Autodesk Inventor part; units mm, degrees
ref_plane "Work Plane1" through (-7.9612, 0, 0) normal (0, -0.866, -0.5) x (1, 0, 0)
ref_plane "YZ Plane" through (0, 0, 0) normal (1, 0, 0) x (0, 1, 0)
ref_plane "XZ Plane" through (0, 0, 0) normal (0, 1, 0) x (-1, 0, 0)
sketch "Sketch1" plane through (0, 0, 0) normal (1, 0, 0) x (0, 1, 0)
  line L0 (-4.0415, 0) -> (-2.0207, 3.5)
  line L1 (-2.0207, 3.5) -> (2.0207, 3.5)
  line L2 (2.0207, 3.5) -> (4.0415, 0)
  line L3 (4.0415, 0) -> (2.0207, -3.5)
  line L4 (2.0207, -3.5) -> (-2.0207, -3.5)
  line L5 (-2.0207, -3.5) -> (-4.0415, 0)
  point P0 (0, 0)
  point P1 (0, 0)
  dimension "d0" = 8.0829
extrude "Body" add sketch "Sketch1" along normal blind 3.2
sketch "Sketch2" plane through (0, 0, 0) normal (0, 0, 1) x (1, 0, 0)
  line L0 (0, 2.0207) -> (0, 4.0415)
  line L1 (0, 4.0415) -> (3.2, 4.0415)
  line L2 (3.2, 2.0207) -> (3.2, 4.0415)
  line L3 (-0.64, 0) -> (3.84, 0)
  line L4 (0.2525, 4.0415) -> (0, 3.5)
  line L5 (2.9475, 4.0415) -> (3.2, 3.5)
  dimension "d3" = 25
  dimension "d4" = 25
  dimension "d5" = 7
  dimension "d6" = 7
revolve "Chamfer1" cut sketch "Sketch2" angle 360 about axis through (-10, 0, 0) along (1, 0, 0)
sketch "Sketch3" plane through (3.2, 0, 0) normal (1, 0, 0) x (0, 0, -1)
  arc A0 (-1.75, -3.0311) -> (1.75, -3.0311) centre (0, 0) ccw
hole "Thread" at (3.2, 0, 0) direction (-1, 0, 0) diameter 3.242 end through all
chamfer "Chamfer2" distance 0.3789 angle 30 1 edges at (3.2, 0, 1.621) measured on face at (3.2, 2.8569, -0.0651)
chamfer "Chamfer3" distance 0.3789 angle 30 1 edges at (0, 0, 1.621) measured on face at (0, 2.8569, -0.0651)
ref_plane "Work Plane1" through (-7.9612, 0, 0) normal (0, -0.866, -0.5) x (1, 0, 0)
equation "\"d0\" = 1.1547 * SW"
equation "\"d1\" = KOH"
equation "\"d8\" = -0.5 * GD1 + 0.5 * NND"
equation "\"d40\" = -0.5 * GD1 + 0.5 * NND"
equation "\"d10\" = -0.5 * GD1 + 0.5 * NND"
equation "\"d41\" = -0.5 * GD1 + 0.5 * NND"
equation "\"d3\" = ANG1"
equation "\"d4\" = ANG2"
equation "\"d5\" = SW0"
equation "\"d6\" = SW01"
equation "\"ANG1\" = 25deg"
equation "\"ANG2\" = 25deg"
equation "\"NND\" = 4"
equation "\"KOH\" = 3.2"
equation "\"SW\" = 7"
equation "\"SW0\" = SW"
equation "\"SW01\" = SW"
equation "\"GUL\" = 0.541266 * PTC"
equation "\"THREADDIA\" = 4"
equation "\"TOA\" = 30deg"
equation "\"PTC\" = 0.7"
equation "\"E0\" = 1.155 * SW"
equation "\"GAL\" = 0.541266 * PTC"
equation "\"SD2\" = 0"
equation "\"WFT\" = 0"
properties part number "ANSI B 18.2.4.1 M - M4 x 0.7" material "Steel, Mild"
CAD build for the part. Positions are in the model's coordinates, mm. Give positions to 0.01 mm unless a question says otherwise; leave off trailing zeros. Order: outer loops, then holes, each group sorted by start corner. A loop starts at its lowest first (then second) coordinate and runs counter-clockwise, first axis right, second up. Notation, with made-up numbers: (54.25, 86) -> (113.25, 86) arc R7 ccw to (113.25, 93) -> close; hole circle Ø10 at (24, 34). An arc over 180 degrees is marked (long way). Return JSON: item names as keys, results as strings.
Q1. Saw through at A-A (x = 2.1). Write the cut outline in (y, z), then the cut area to 3 significant figures.
Working result:
{"outline": "(-4.04, 0) -> (-2.02, -3.5) -> (2.02, -3.5) -> (4.04, 0) -> (2.02, 3.5) -> (-2.02, 3.5) -> close; hole circle Ø3.24 at (0, 0)", "area": "34.2 mm²"}
Q2. Mould opens along Z. For faces 1 (the face through (1.581, 1.438, -0.748)), 2 (the face through (0.089, -1.854, -3.193)), 3 (the face through (3.11, 3.69, 0.01)), 4 (the face through (1.578, -3.045, 1.726)) say: pulls with the +Z half, pulls with the -Z half, needs draft (parallel to the pull), parting line crosses it, or undercut.
Working result:
{"face 1": "undercut", "face 2": "pulls with the -Z half", "face 3": "parting line crosses it", "face 4": "pulls with the +Z half"}
Q3. Drill centre lines: line 1 (Z direction, x = 1.2, y = 0); line 2 (Y direction, x = 2.25, z = 1.75); line 3 (Y direction, x = 1.6, z = -0.25). Where is each one in solid material? Low to high.
Working result:
{"line 1": "-3.5 to -1.62, 1.62 to 3.5", "line 2": "-3.03 to 3.03", "line 3": "-3.9 to -1.6, 1.6 to 3.9"}
Q4. Flat gauge pins, fed straight in: pin 1 (1 mm diameter, centred on x = 2, z = 2, fed in from -Y); pin 2 (4 mm diameter, centred on y = 2.5, z = -2.5, fed in from +X). Where does each tip first touch, or does it go through?
Working result:
{"pin 1": "y = -3.18", "pin 2": "x = 3.2"}
